Build history of the part. All positions in model axes, mm. Face numbers are marked on the shaded views. A direction names the side the tool comes from. Coordinates: 2 decimals unless noted, no trailing zeros. Write each loop counter-clockwise with the first axis right and the second up, starting at its lowest first coordinate (ties: lowest second). Pieces come first, ordered by that corner, then holes.
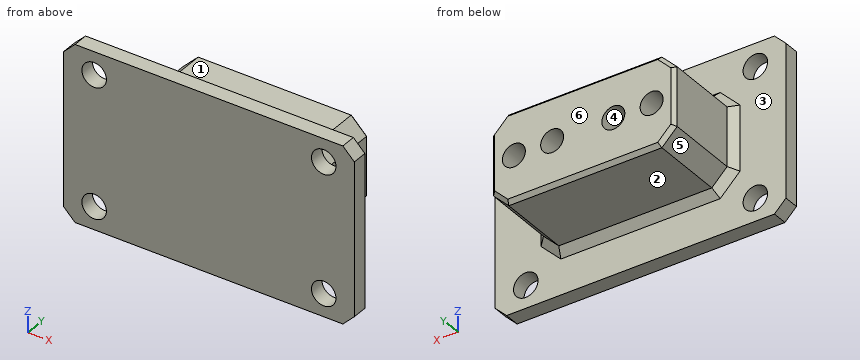
```python
from build123d import *

# Parameters (mm, degrees)
SKETCH1_W           = 38
SKETCH1_H           = 23
SKETCH1_R           = 1.6
BOSS_EXTRUDE1_DEPTH = 2
SKETCH2_W           = 24
SKETCH2_H           = 11.708497378
SKETCH2_R           = 1.5
BOSS_EXTRUDE2_DEPTH = 11
CHAMFER1_SIZE       = 2
CHAMFER2_SIZE       = 1
CHAMFER3_SIZE       = 1.5
CHAMFER4_SIZE       = 0.5


with BuildPart() as part:
    # Sketch1 → Boss-Extrude1 (new body)
    with BuildSketch(Plane(origin=(0, 0, 0), x_dir=(1, 0, 0), z_dir=(0, 1, 0))):
        Rectangle(SKETCH1_W, SKETCH1_H)
        with Locations(Location((-15, 8.5, 0), (0, 0, 270))):
            Circle(SKETCH1_R, mode=Mode.SUBTRACT)
        with Locations(Location((15, 8.5, 0), (0, 0, 90))):
            Circle(SKETCH1_R, mode=Mode.SUBTRACT)
        with Locations(Location((15, -8.5, 0), (0, 0, 270))):
            Circle(SKETCH1_R, mode=Mode.SUBTRACT)
        with Locations(Location((-15, -8.5, 0), (0, 0, 90))):
            Circle(SKETCH1_R, mode=Mode.SUBTRACT)
    extrude(amount=BOSS_EXTRUDE1_DEPTH)

    # Sketch2 → Boss-Extrude2 (add)
    with BuildSketch(Plane(origin=(0, 2, 0), x_dir=(1, 0, 0), z_dir=(0, 1, 0))):
        Rectangle(SKETCH2_W, SKETCH2_H)
        with Locations(Location((-9, 0, 0), (0, 0, 270))):
            Circle(SKETCH2_R, mode=Mode.SUBTRACT)
        with Locations(Location((-4, 0, 0), (0, 0, 270))):
            Circle(SKETCH2_R, mode=Mode.SUBTRACT)
        with Locations(Location((4, 0, 0), (0, 0, 90))):
            Circle(SKETCH2_R, mode=Mode.SUBTRACT)
        with Locations(Location((9, 0, 0), (0, 0, 90))):
            Circle(SKETCH2_R, mode=Mode.SUBTRACT)
    extrude(amount=BOSS_EXTRUDE2_DEPTH)

    # Chamfer1
    chamfer1_edges = [part.edges().sort_by_distance(p)[0] for p in [
        (12, 7.5, 5.854248689),
        (12, 7.5, -5.854248689),
        (-12, 7.5, -5.854248689),
        (-12, 7.5, 5.854248689),
    ]]
    chamfer(chamfer1_edges, length=CHAMFER1_SIZE)

    # Chamfer2
    chamfer2_edges = [part.edges().sort_by_distance(p)[0] for p in [
        (0, 2, 5.854248689),
        (-12, 2, 0),
        (0, 2, -5.854248689),
        (12, 2, 0),
        (-11, 2, 4.854248689),
        (-11, 2, -4.854248689),
        (11, 2, -4.854248689),
        (11, 2, 4.854248689),
    ]]
    chamfer(chamfer2_edges, length=CHAMFER2_SIZE)

    # Chamfer3
    chamfer3_edges = [part.edges().sort_by_distance(p)[0] for p in [
        (19, 1, 11.5),
        (-19, 1, 11.5),
        (-19, 1, -11.5),
        (19, 1, -11.5),
    ]]
    chamfer(chamfer3_edges, length=CHAMFER3_SIZE)

    # Chamfer4
    chamfer4_edges = [part.edges().sort_by_distance(p)[0] for p in [
        (0, 13, 5.854248689),
        (-12, 13, 0),
        (12, 13, 0),
        (0, 13, -5.854248689),
        (11, 13, 4.854248689),
        (11, 13, -4.854248689),
        (-11, 13, -4.854248689),
        (-11, 13, 4.854248689),
    ]]
    chamfer(chamfer4_edges, length=CHAMFER4_SIZE)


solid = part.part
```
1. Flat gauge pins, fed straight in: pin 1 (0.9 mm diameter, centred on x = 9.5, z = 0.5, fed in from +Y); pin 2 (2 mm diameter, centred on y = 8, z = 2.5, fed in from -X); pin 3 (1.5 mm diameter, centred on y = 5, z = 0, fed in from +X); pin 4 (12 mm diameter, centred on x = -2, z = 8.5, fed in from +Y). Where does each tip first touch, or does it go through?
Computed values:
pin 1: stops at y = 2
pin 2: stops at x = -12
pin 3: stops at x = 12
pin 4: stops at y = 13
2. Saw through at A-A on x = -15. List the corners of the cut face in (y, z), plus the area to 3 significant figures.
Computed values:
outline: (0, -11.5) - (2, -11.5) - (2, -10.1) - (0, -10.1) - close; (0, -6.9) - (2, -6.9) - (2, 6.9) - (0, 6.9) - close; (0, 10.1) - (2, 10.1) - (2, 11.5) - (0, 11.5) - close
area: 33.2 mm2
3. 3-axis set-ups, long thin cutter, end or side, ignore diameter. For the marked faces 1, 2 and 3: which of +Z, -Z, +X, -X, +Y, -Y reach the whole face in a straight line?
Computed values:
face 1: +Z, +X, -X, +Y
face 2: -Z, +X, -X, +Y
face 3: +Y
4. Probe line 1 along X through (y, z) = (1, 8.5); line 2 along X through (y, z) = (8.5, 0); line 3 along Y through (x, z) = (16, -2.75). List the from-to ranges inside material, lowest first.
Computed values:
line 1: x = -19 to -16.6, -13.4 to 13.4, 16.6 to 19
line 2: x = -12 to -10.5, -7.5 to -5.5, -2.5 to 2.5, 5.5 to 7.5, 10.5 to 12
line 3: y = 0 to 2
5. Saw through at B-B on z = -8.5. List the corners of the cut face in (x, y), plus the area to 3 significant figures.
Computed values:
outline: (-19, 0) - (-16.6, 0) - (-16.6, 2) - (-19, 2) - close; (-13.4, 0) - (13.4, 0) - (13.4, 2) - (-13.4, 2) - close; (16.6, 0) - (19, 0) - (19, 2) - (16.6, 2) - close
area: 63.2 mm2
6. Saw through at C-C on y = 8.75. List the corners of the cut face in (x, z).
Computed values:
outline: (-12, -3.85) - (-10, -5.85) - (10, -5.85) - (12, -3.85) - (12, 3.85) - (10, 5.85) - (-10, 5.85) - (-12, 3.85) - close; hole circle Ø3 at (-9, 0); hole circle Ø3 at (-4, 0); hole circle Ø3 at (4, 0); hole circle Ø3 at (9, 0)
7. Saw through at D-D on x = 0.5. List the corners of the cut face in (y, z).
Computed values:
outline: (0, -11.5) - (2, -11.5) - (2, -6.85) - (3, -5.85) - (12.5, -5.85) - (13, -5.35) - (13, 5.35) - (12.5, 5.85) - (3, 5.85) - (2, 6.85) - (2, 11.5) - (0, 11.5) - close
8. Mould opens along X. For the marked faces 4, 5 and 6 say: +X half, -X half, draft (parallel to the pull), parting line (faces both ways), or undercut.
Computed values:
face 4: undercut
face 5: -X half
face 6: draft
